CAD build for the part. Positions are in the model's coordinates, mm. Face numbers are marked on the shaded views. A direction names the side the tool comes from. Round coordinates to 2 decimals unless told otherwise and drop trailing zeros. Order: outer loops, then holes, each group sorted by start corner. A loop starts at its lowest first (then second) coordinate and runs counter-clockwise, first axis right, second up. Notation, with made-up numbers: (4.25, -17.5) -> (50.25, -17.5) arc R22 ccw to (50.25, 15.5) -> close; hole circle Ø8 at (-26.75, 87.5). An arc over 180 degrees is marked (long way). Return JSON: item names as keys, results as strings. Group by question number.
Q1. Probe line 1 along Z through (x, y) = (28.5, 56); line 2 along X through (y, z) = (58, 342); line 3 along Y through (x, z) = (195, 185). List the from-to ranges inside material, lowest first.
Q2. Cut at D-D (z = 254). Write the cut outline in (x, y), then the cut area to 3 significant figures.
Q3. Cut at C-C (x = 163). Write the cut outline in (y, z).
Q4. Which spindle directions (+Z, -Z, +X, -X, +Y, -Y) get a long thin tool onto all of the face, cutting with end or side? Do the marked faces 1, 2 and 3. Say none if no direction does.
Q5. Cut at B-B (y = 32). Write the cut outline in (x, z).
Q6. Flat gauge pins, fed straight in: pin 1 (0.5 mm diameter, centred on y = 62.5, z = 244.5, fed in from +X); pin 2 (0.8 mm diameter, centred on x = 61, z = 380, fed in from -Y); pin 3 (5 mm diameter, centred on y = 44.45, z = 330.2, fed in from +X). Where does each tip first touch, or does it go through?
Q7. Cut at A-A (x = 52.5). Write the cut outline in (y, z).
Q8. Mould opens along X. For the marked faces 4, 5 and 6 say: +X half, -X half, draft (parallel to the pull), parting line (faces both ways), or undercut.
from build123d import *

# Parameters (mm, degrees)
BOSS_EXTRUDE1_DEPTH = 381
CUT_EXTRUDE1_DEPTH  = 304.8
SHELL1_T            = -2.54
SKETCH4_W           = 121.92
SKETCH4_H           = 50.8
CUT_EXTRUDE3_DEPTH  = 2.54
CUT_EXTRUDE4_START  = -381
SKETCH4_4_W         = 121.92
SKETCH4_4_H         = 50.8
CUT_EXTRUDE4_DEPTH  = 2.54
SKETCH5_R           = 3.175
CUT_EXTRUDE5_DEPTH  = 2.54
BOSS_EXTRUDE2_START = 63.5
SKETCH7_W           = 196.692393165
SKETCH7_H           = 375.92
BOSS_EXTRUDE2_DEPTH = 1.5875
SKETCH8_R           = 2.667
CUT_EXTRUDE6_DEPTH  = 2.54


with BuildPart() as part:
    # Sketch2 → Boss-Extrude1 (new body)
    with BuildSketch(Plane.XY):
        Polygon((0, 0), (127, 0), (203.2, 63.5), (0, 63.5), align=None)
    extrude(amount=BOSS_EXTRUDE1_DEPTH)

    # Sketch3 → Cut-Extrude1 (cut)
    with BuildSketch(Plane.ZY):
        Polygon((0, 0), (381, 0), (190.5, 50.8), align=None)
    extrude(amount=-CUT_EXTRUDE1_DEPTH, mode=Mode.SUBTRACT)

    # Shell1
    shell1_openings = [part.faces().sort_by_distance(p)[0] for p in [
        (101.6, 63.5, 190.5),
    ]]
    offset(amount=SHELL1_T, openings=shell1_openings, kind=Kind.INTERSECTION)

    # Sketch4 → Cut-Extrude3 (cut)
    with BuildSketch(Plane.XY.offset(381)):
        with Locations((63.5, 28.956)):
            Rectangle(SKETCH4_W, SKETCH4_H)
    extrude(amount=-CUT_EXTRUDE3_DEPTH, mode=Mode.SUBTRACT)

    # Sketch4<4> → Cut-Extrude4 (cut)
    with BuildSketch(Plane.XY.offset(381).offset(CUT_EXTRUDE4_START)):
        with Locations((63.5, 28.956)):
            Rectangle(SKETCH4_4_W, SKETCH4_4_H)
    extrude(amount=CUT_EXTRUDE4_DEPTH, mode=Mode.SUBTRACT)

    # Sketch5 → Cut-Extrude5 (cut)
    with BuildSketch(Plane(origin=(0, 94.854771784, 25.294605809), x_dir=(1, 0, 0), z_dir=(0, -0.9662349396012463, -0.2576626505603321))):
        with Locations(Location((31.75, 355.435511988, 0), (0, 0, 270))):
            Circle(SKETCH5_R)
        with Locations(Location((95.25, 355.435511988, 0), (0, 0, 270))):
            Circle(SKETCH5_R)
    cut_extrude5 = extrude(amount=-CUT_EXTRUDE5_DEPTH, mode=Mode.SUBTRACT)

    # Mirror1: Cut-Extrude5 across plane
    add(cut_extrude5.mirror(Plane.XY.offset(190.5)), mode=Mode.SUBTRACT)

    # Sketch7 → Boss-Extrude2 (add)
    with BuildSketch(Plane(origin=(0, 0, 0), x_dir=(1, 0, 0), z_dir=(0, 1, 0)).offset(BOSS_EXTRUDE2_START)):
        with Locations((100.886196583, -190.5)):
            Rectangle(SKETCH7_W, SKETCH7_H)
        Polygon((8.89, -372.11), (126.999705463, -372.11), (192.882393165, -372.11), (192.882393165, -8.89), (126.999705463, -8.89), (8.89, -8.89), (8.89, -190.5), align=None, mode=Mode.SUBTRACT)
    extrude(amount=-BOSS_EXTRUDE2_DEPTH)

    # Sketch8 → Cut-Extrude6 (cut)
    with BuildSketch(Plane.ZY):
        with Locations(Location((309.626, 44.45, 0), (0, 0, 270))):
            Circle(SKETCH8_R)
        with Locations(Location((330.2, 44.45, 0), (0, 0, 270))):
            Circle(SKETCH8_R)
    cut_extrude6 = extrude(amount=-CUT_EXTRUDE6_DEPTH, mode=Mode.SUBTRACT)

    # Mirror2: Cut-Extrude6 across plane
    add(cut_extrude6.mirror(Plane.XY.offset(190.5)), mode=Mode.SUBTRACT)


solid = part.part
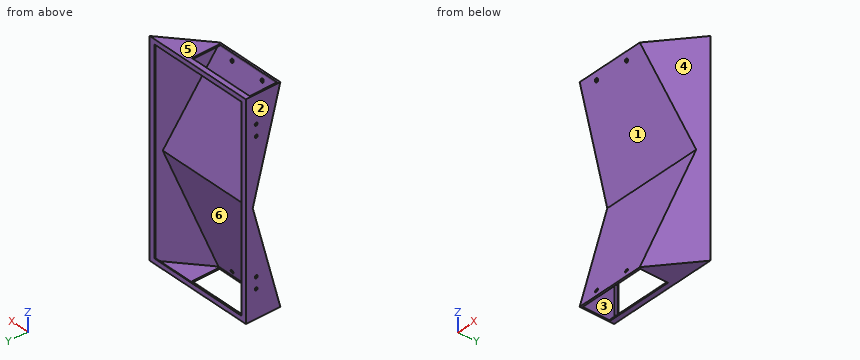
Solution:
{
 "1": {"line 1": "z = 0 to 2.54, 378.46 to 381", "line 2": "x = 0 to 2.54, 192.63 to 196.6", "line 3": "y = 56.67 to 59.97, 61.91 to 63.5"},
 "2": {"outline": "(0, 33.87) -> (167.64, 33.87) -> (203.2, 63.5) -> (192.88, 63.5) -> (192.88, 61.91) -> (197.33, 61.91) -> (166.83, 36.5) -> (2.54, 36.5) -> (2.54, 61.91) -> (8.89, 61.91) -> (8.89, 63.5) -> (0, 63.5) -> close", "area": "639 mm²"},
 "3": {"outline": "(30, 0) -> (63.5, 0) -> (63.5, 8.89) -> (61.91, 8.89) -> (61.91, 2.54) -> (33.31, 2.54) -> (33.31, 115.04) -> (53.43, 190.5) -> (33.31, 265.96) -> (33.31, 378.46) -> (61.91, 378.46) -> (61.91, 372.11) -> (63.5, 372.11) -> (63.5, 381) -> (30, 381) -> (30, 268.5) -> (50.8, 190.5) -> (30, 112.5) -> close"},
 "4": {"face 1": "+X, -X, -Y", "face 2": "+Z, -Z, -X, +Y, -Y", "face 3": "none"},
 "5": {"outline": "(0, 0) -> (2.54, 0) -> (2.54, 110.14) -> (161.43, 110.14) -> (161.43, 2.54) -> (124.46, 2.54) -> (124.46, 0) -> (165.4, 0) -> (165.4, 120) -> (0, 120) -> close; (0, 261) -> (165.4, 261) -> (165.4, 381) -> (124.46, 381) -> (124.46, 378.46) -> (161.43, 378.46) -> (161.43, 270.86) -> (2.54, 270.86) -> (2.54, 381) -> (0, 381) -> close"},
 "6": {"pin 1": "stops at x = 202.3", "pin 2": "stops at y = 0.16", "pin 3": "stops at x = 183.34"},
 "7": {"outline": "(0, 0) -> (3.56, 0) -> (3.56, 2.54) -> (3.31, 2.54) -> (53.43, 190.5) -> (3.31, 378.46) -> (3.56, 378.46) -> (3.56, 381) -> (0, 381) -> (50.8, 190.5) -> close; (54.36, 0) -> (63.5, 0) -> (63.5, 8.89) -> (61.91, 8.89) -> (61.91, 2.54) -> (54.36, 2.54) -> close; (54.36, 378.46) -> (61.91, 378.46) -> (61.91, 372.11) -> (63.5, 372.11) -> (63.5, 381) -> (54.36, 381) -> close"},
 "8": {"face 4": "+X half", "face 5": "draft", "face 6": "undercut"}
}
